The drawing under review shows one solid part. Ordinate dimensions are in mm from its lowest x, y, z. A direction names the side the tool comes from. Give positions to 0.01 mm unless a question says otherwise; leave off trailing zeros. Order: outer loops, then holes, each group sorted by start corner. A loop starts at its lowest first (then second) coordinate and runs counter-clockwise, first axis right, second up. Notation, with made-up numbers: (72.5, 78.25) - (91.5, 78.25) arc R24 cw to (91.5, 93.25) - close; hole circle Ø7 at (32, -16.75). An arc over 180 degrees is marked (long way). Write item = value, one per line. Start each with the question number.
1. Mouldability with a two-part tool opening along X and no side actions: class the marked faces 3, 4, 5 and 6 as pulls with the +X half, pulls with the -X half, needs draft (parallel to the pull), parting line crosses it, or undercut.
2. We need section A-A, the plane z = 14. Give the boundary of the cut face in (x, y) (1 decimal).
3. Machinability: for the marked faces 1 and 2, which of the approach directions +Z, -Z, +X, -X, +Y, -Y give a long, thin tool a straight path to every point of the face, cutting with its end or side? Answer none if there is none.
4. Wall thickness on probe 1 along X at (y, z) = (24, 2.55); probe 2 along Y at (x, z) = (14.75, 2.3); probe 3 along X at (y, z) = (13.5, 10.25): over which ranges is each line inside the solid? List them lowest first.
5. We need section B-B, the plane x = 6.5. Give the boundary of the cut face in (y, z), and give its area (3 significant figures).
6. For P1, Ø5.5, axis at x = 23, y = 24, coming from the +Z side; P2, Ø8, axis at x = 14.71, z = 14, coming from the +Y side, all flat-tipped, find the tip position at first contact; note any pin that passes through.
7. We need section D-D, the plane y = 8. Give the boundary of the cut face in (x, z).
8. We need section C-C, the plane y = 24. Give the boundary of the cut face in (x, z).
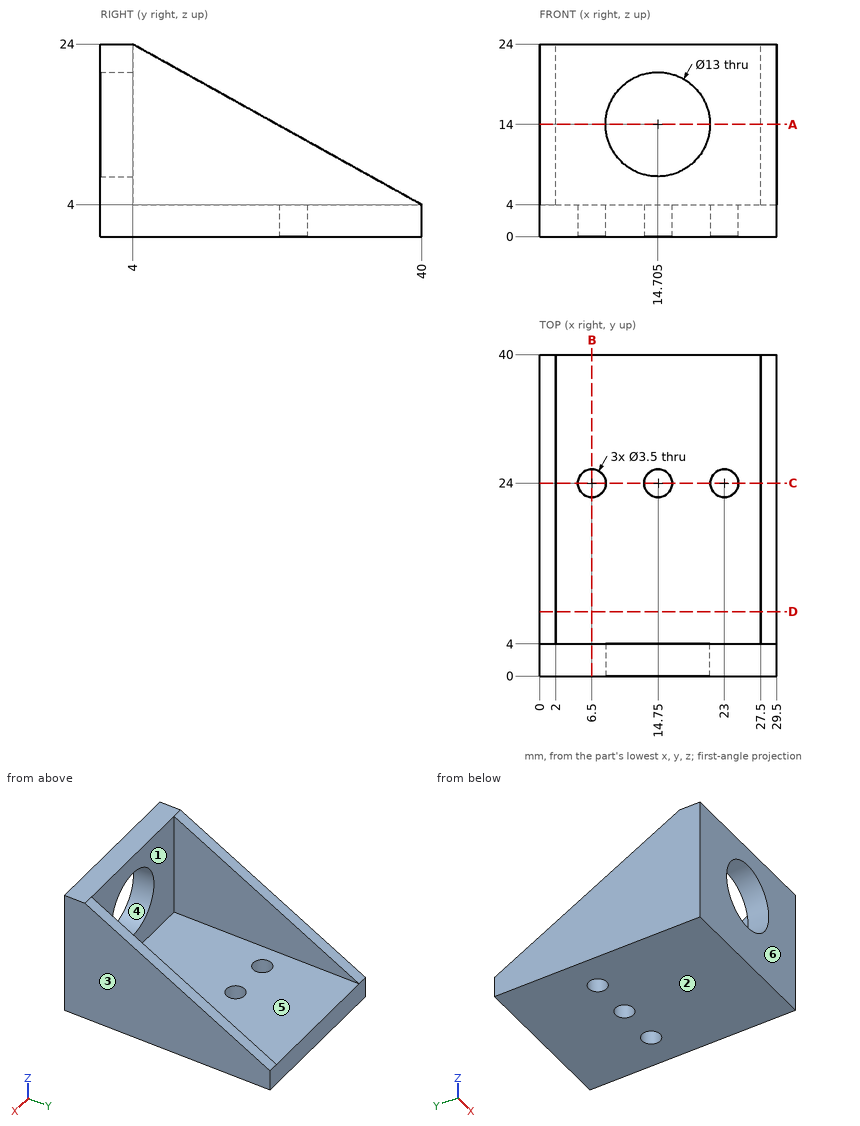
Model answer:
q1.face_3 = pulls with the +X half
q1.face_4 = undercut
q1.face_5 = undercut
q1.face_6 = needs draft
q2.outline = (0, 0) - (8.2, 0) - (8.2, 4) - (2, 4) - (2, 22) - (0, 22) - close; (21.2, 0) - (29.5, 0) - (29.5, 22) - (27.5, 22) - (27.5, 4) - (21.2, 4) - close
q3.face_1 = +Z, +Y
q3.face_2 = -Z, +X, -X, +Y, -Y
q4.probe_1 = 0 to 4.75, 8.25 to 13, 16.5 to 21.25, 24.75 to 29.5
q4.probe_2 = 0 to 22.25, 25.75 to 40
q4.probe_3 = 0 to 2, 27.5 to 29.5
q5.outline = (0, 0) - (22.25, 0) - (22.25, 4) - (4, 4) - (4, 24) - (0, 24) - close; (25.75, 0) - (40, 0) - (40, 4) - (25.75, 4) - close
q5.area = 226 mm2
q6.P1 = 4
q6.P2 = through
q7.outline = (0, 0) - (29.5, 0) - (29.5, 21.78) - (27.5, 21.78) - (27.5, 4) - (2, 4) - (2, 21.78) - (0, 21.78) - close
q8.outline = (0, 0) - (4.75, 0) - (4.75, 4) - (2, 4) - (2, 12.89) - (0, 12.89) - close; (8.25, 0) - (13, 0) - (13, 4) - (8.25, 4) - close; (16.5, 0) - (21.25, 0) - (21.25, 4) - (16.5, 4) - close; (24.75, 0) - (29.5, 0) - (29.5, 12.89) - (27.5, 12.89) - (27.5, 4) - (24.75, 4) - close
